Geometry check sheet. Reference: drawing and pictorial views, mm from the part's lowest x, y, z. Coordinates: 2 decimals unless noted, no trailing zeros. Write each loop counter-clockwise with the first axis right and the second up, starting at its lowest first coordinate (ties: lowest second). Pieces come first, ordered by that corner, then holes. Notation, with made-up numbers: (9, -32.5) - (58, -32.5) arc R23 ccw to (58, -20.5) - close; hole circle Ø8 at (-17.75, -34). An arc over 180 degrees is marked (long way). Answer as a JSON object with one key per item and string values. Group by question number.
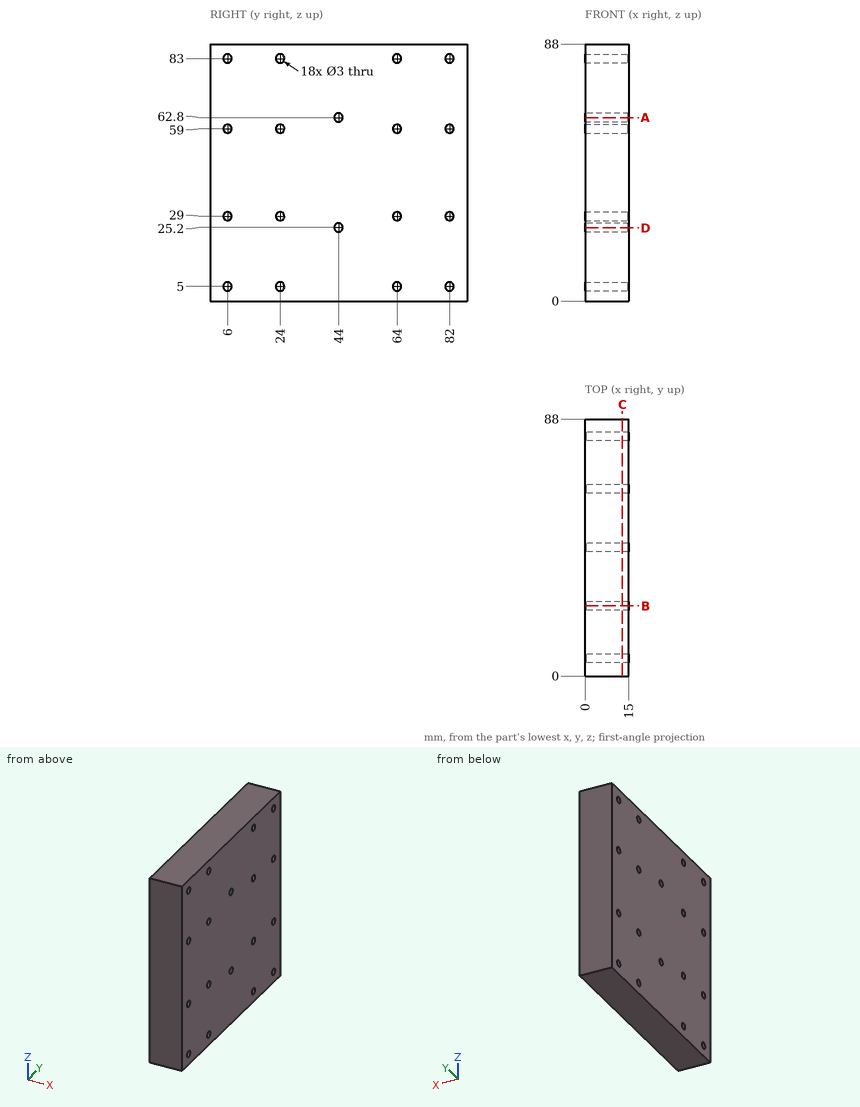
(1) Section check A-A (z = 62.8). Record the cut outline in (x, y), and give its area (4 significant figures).
(2) Section check D-D (z = 25). Record the cut outline in (x, y), and give its area (3 significant figures).
(3) Section check B-B (y = 24). Record the cut outline in (x, z), and give its area (3 significant figures).
(4) Material ranges on L1, parallel to Z at x = 8.5, y = 64; L2, parallel to Y at x = 11.75, z = 83; L3, parallel to Y at x = 10, z = 58, recorded low to high. Write a range as [from, to].
(5) Gauge pin test, flat end, axial feed: pin 1 (3 mm diameter, centred on x = 7.5, y = 77, fed in from -Z). Record the tip position at first contact, or that the pin passes through.
(6) Section check C-C (x = 12.75). Count the separate pieces of the cut face and the enclosed holes in it, and give its area (3 significant figures).
Conclusion:
{
 "1": {"outline": "(0, 0) - (15, 0) - (15, 42.5) - (0, 42.5) - close; (0, 45.5) - (15, 45.5) - (15, 88) - (0, 88) - close", "area": "1,275 mm^2"},
 "2": {"outline": "(0, 0) - (15, 0) - (15, 42.51) - (0, 42.51) - close; (0, 45.49) - (15, 45.49) - (15, 88) - (0, 88) - close", "area": "1,280 mm^2"},
 "3": {"outline": "(0, 0) - (15, 0) - (15, 3.5) - (0, 3.5) - close; (0, 6.5) - (15, 6.5) - (15, 27.5) - (0, 27.5) - close; (0, 30.5) - (15, 30.5) - (15, 57.5) - (0, 57.5) - close; (0, 60.5) - (15, 60.5) - (15, 81.5) - (0, 81.5) - close; (0, 84.5) - (15, 84.5) - (15, 88) - (0, 88) - close", "area": "1,140 mm^2"},
 "4": {"L1": "z = [0, 3.5], [6.5, 27.5], [30.5, 57.5], [60.5, 81.5], [84.5, 88]", "L2": "y = [0, 4.5], [7.5, 22.5], [25.5, 62.5], [65.5, 80.5], [83.5, 88]", "L3": "y = [0, 4.88], [7.12, 22.88], [25.12, 62.88], [65.12, 80.88], [83.12, 88]"},
 "5": {"pin 1": "stops at z = 0"},
 "6": {"separate pieces": "1", "enclosed holes": "18", "area": "7,620 mm^2"}
}
